For this review, take the finished solid that the model builds, in its own axes (mm). Face numbers are marked on the shaded views. A direction names the side the tool comes from. Round coordinates to 2 decimals unless told otherwise and drop trailing zeros. Order: outer loops, then holes, each group sorted by start corner. A loop starts at its lowest first (then second) coordinate and runs counter-clockwise, first axis right, second up.
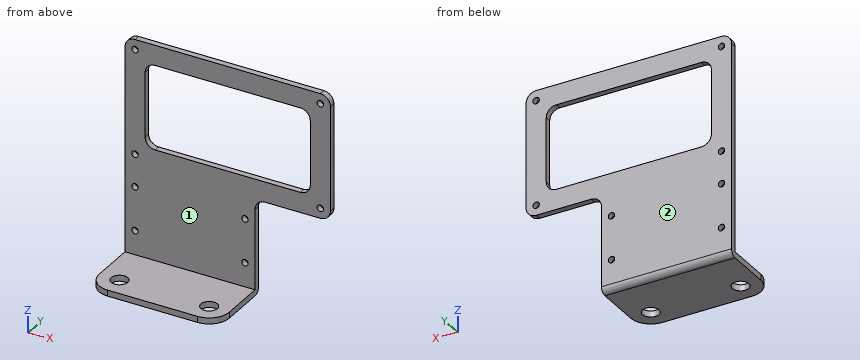
```python
from build123d import *

# Parameters (mm, degrees)
SKETCH_1_W          = 110
SKETCH_1_H          = 110
EXTRUDE_1_DEPTH     = 3
CUT_EXTRUDE_1_REACH = 79.84
SKETCH_2_R          = 1.6
CUT_EXTRUDE_2_REACH = 79.84
SKETCH_5_W          = 64.6
SKETCH_5_H          = 3
EXTRUDE_2_DEPTH     = 32
CUT_EXTRUDE_3_REACH = 129.079
SKETCH_6_R          = 4.1
CUT_EXTRUDE_4_REACH = 87.294
FILLET_1_R          = 5
FILLET_2_R          = 3
FILLET_3_R          = 10


with BuildPart() as part:
    # 草图1 → 凸台-拉伸1 (new body)
    with BuildSketch(Plane(origin=(0, 0, 0), x_dir=(1, 0, 0), z_dir=(0, 1, 0))):
        Rectangle(SKETCH_1_W, SKETCH_1_H)
    extrude(amount=EXTRUDE_1_DEPTH)

    # 草图2 → 切除-拉伸1 (cut, up to next)
    with BuildSketch(Plane(origin=(0, 3, 0), x_dir=(1, 0, 0), z_dir=(0, 1, 0)), mode=Mode.PRIVATE) as cut_extrude_1_sk1:
        with Locations(Location((-50, 40, 0), (0, 0, 270))):
            Circle(SKETCH_2_R)
    cut_extrude_1_tool1 = extrude(cut_extrude_1_sk1.sketch, amount=-CUT_EXTRUDE_1_REACH, mode=Mode.PRIVATE) & part.part
    # 草图2 → 切除-拉伸1 (cut, up to next)
    with BuildSketch(Plane(origin=(0, 3, 0), x_dir=(1, 0, 0), z_dir=(0, 1, 0)), mode=Mode.PRIVATE) as cut_extrude_1_sk2:
        with Locations(Location((4.6, 40, 0), (0, 0, 270))):
            Circle(SKETCH_2_R)
    cut_extrude_1_tool2 = extrude(cut_extrude_1_sk2.sketch, amount=-CUT_EXTRUDE_1_REACH, mode=Mode.PRIVATE) & part.part
    # 草图2 → 切除-拉伸1 (cut, up to next)
    with BuildSketch(Plane(origin=(0, 3, 0), x_dir=(1, 0, 0), z_dir=(0, 1, 0)), mode=Mode.PRIVATE) as cut_extrude_1_sk3:
        with Locations(Location((4.6, 18.2, 0), (0, 0, 270))):
            Circle(SKETCH_2_R)
    cut_extrude_1_tool3 = extrude(cut_extrude_1_sk3.sketch, amount=-CUT_EXTRUDE_1_REACH, mode=Mode.PRIVATE) & part.part
    # 草图2 → 切除-拉伸1 (cut, up to next)
    with BuildSketch(Plane(origin=(0, 3, 0), x_dir=(1, 0, 0), z_dir=(0, 1, 0)), mode=Mode.PRIVATE) as cut_extrude_1_sk4:
        with Locations(Location((-50, 18.2, 0), (0, 0, 270))):
            Circle(SKETCH_2_R)
    cut_extrude_1_tool4 = extrude(cut_extrude_1_sk4.sketch, amount=-CUT_EXTRUDE_1_REACH, mode=Mode.PRIVATE) & part.part
    # 草图2 → 切除-拉伸1 (cut, up to next)
    with BuildSketch(Plane(origin=(0, 3, 0), x_dir=(1, 0, 0), z_dir=(0, 1, 0)), mode=Mode.PRIVATE) as cut_extrude_1_sk5:
        with Locations(Location((-50, -50, 0), (0, 0, 270))):
            Circle(SKETCH_2_R)
    cut_extrude_1_tool5 = extrude(cut_extrude_1_sk5.sketch, amount=-CUT_EXTRUDE_1_REACH, mode=Mode.PRIVATE) & part.part
    # 草图2 → 切除-拉伸1 (cut, up to next)
    with BuildSketch(Plane(origin=(0, 3, 0), x_dir=(1, 0, 0), z_dir=(0, 1, 0)), mode=Mode.PRIVATE) as cut_extrude_1_sk6:
        with Locations(Location((42, -50, 0), (0, 0, 270))):
            Circle(SKETCH_2_R)
    cut_extrude_1_tool6 = extrude(cut_extrude_1_sk6.sketch, amount=-CUT_EXTRUDE_1_REACH, mode=Mode.PRIVATE) & part.part
    # 草图2 → 切除-拉伸1 (cut, up to next)
    with BuildSketch(Plane(origin=(0, 3, 0), x_dir=(1, 0, 0), z_dir=(0, 1, 0)), mode=Mode.PRIVATE) as cut_extrude_1_sk7:
        with Locations(Location((42, 2, 0), (0, 0, 270))):
            Circle(SKETCH_2_R)
    cut_extrude_1_tool7 = extrude(cut_extrude_1_sk7.sketch, amount=-CUT_EXTRUDE_1_REACH, mode=Mode.PRIVATE) & part.part
    # 草图2 → 切除-拉伸1 (cut, up to next)
    with BuildSketch(Plane(origin=(0, 3, 0), x_dir=(1, 0, 0), z_dir=(0, 1, 0)), mode=Mode.PRIVATE) as cut_extrude_1_sk8:
        with Locations(Location((-50, 2, 0), (0, 0, 270))):
            Circle(SKETCH_2_R)
    cut_extrude_1_tool8 = extrude(cut_extrude_1_sk8.sketch, amount=-CUT_EXTRUDE_1_REACH, mode=Mode.PRIVATE) & part.part
    add(cut_extrude_1_tool1.solids().sort_by_distance((-50, 3, -40))[0], mode=Mode.SUBTRACT)
    add(cut_extrude_1_tool2.solids().sort_by_distance((4.6, 3, -40))[0], mode=Mode.SUBTRACT)
    add(cut_extrude_1_tool3.solids().sort_by_distance((4.6, 3, -18.2))[0], mode=Mode.SUBTRACT)
    add(cut_extrude_1_tool4.solids().sort_by_distance((-50, 3, -18.2))[0], mode=Mode.SUBTRACT)
    add(cut_extrude_1_tool5.solids().sort_by_distance((-50, 3, 50))[0], mode=Mode.SUBTRACT)
    add(cut_extrude_1_tool6.solids().sort_by_distance((42, 3, 50))[0], mode=Mode.SUBTRACT)
    add(cut_extrude_1_tool7.solids().sort_by_distance((42, 3, -2))[0], mode=Mode.SUBTRACT)
    add(cut_extrude_1_tool8.solids().sort_by_distance((-50, 3, -2))[0], mode=Mode.SUBTRACT)

    # 草图3 → 切除-拉伸2 (cut, up to next)
    with BuildSketch(Plane(origin=(0, 3, 0), x_dir=(1, 0, 0), z_dir=(0, 1, 0)), mode=Mode.PRIVATE) as cut_extrude_2_sk1:
        Polygon((55, 17), (55, -55), (47, -55), (47, 7), (9.6, 7), (9.6, 55), (55, 55), align=None)
    cut_extrude_2_tool1 = extrude(cut_extrude_2_sk1.sketch, amount=-CUT_EXTRUDE_2_REACH, mode=Mode.PRIVATE) & part.part
    add(cut_extrude_2_tool1.solids().sort_by_distance((35.767105, 3, -20.802632))[0], mode=Mode.SUBTRACT)

    # 草图5 → 凸台-拉伸2 (add)
    with BuildSketch(Plane.XZ):
        with Locations((-22.7, -53.5)):
            Rectangle(SKETCH_5_W, SKETCH_5_H)
    extrude(amount=EXTRUDE_2_DEPTH)

    # 草图6 → 切除-拉伸3 (cut, up to next)
    with BuildSketch(Plane(origin=(0, 0, -55), x_dir=(-1, 0, 0), z_dir=(0, 0, -1)), mode=Mode.PRIVATE) as cut_extrude_3_sk1:
        with Locations((0.4, -22)):
            Circle(SKETCH_6_R)
    cut_extrude_3_tool1 = extrude(cut_extrude_3_sk1.sketch, amount=-CUT_EXTRUDE_3_REACH, mode=Mode.PRIVATE) & part.part
    # 草图6 → 切除-拉伸3 (cut, up to next)
    with BuildSketch(Plane(origin=(0, 0, -55), x_dir=(-1, 0, 0), z_dir=(0, 0, -1)), mode=Mode.PRIVATE) as cut_extrude_3_sk2:
        with Locations((45, -22)):
            Circle(SKETCH_6_R)
    cut_extrude_3_tool2 = extrude(cut_extrude_3_sk2.sketch, amount=-CUT_EXTRUDE_3_REACH, mode=Mode.PRIVATE) & part.part
    add(cut_extrude_3_tool1.solids().sort_by_distance((-0.4, -22, -55))[0], mode=Mode.SUBTRACT)
    add(cut_extrude_3_tool2.solids().sort_by_distance((-45, -22, -55))[0], mode=Mode.SUBTRACT)

    # 草图7 → 切除-拉伸4 (cut, up to next)
    with BuildSketch(Plane(origin=(0, 3, 0), x_dir=(1, 0, 0), z_dir=(0, 1, 0)), mode=Mode.PRIVATE) as cut_extrude_4_sk1:
        with BuildLine():
            Line((-40, -3), (32, -3))
            ThreePointArc((32, -3), (35.535533906, -4.464466094), (37, -8))
            Line((37, -8), (37, -40))
            ThreePointArc((37, -40), (35.535533906, -43.535533906), (32, -45))
            Line((32, -45), (-40, -45))
            ThreePointArc((-40, -45), (-43.535533906, -43.535533906), (-45, -40))
            Line((-45, -40), (-45, -8))
            ThreePointArc((-45, -8), (-43.535533906, -4.464466094), (-40, -3))
        make_face()
    cut_extrude_4_tool1 = extrude(cut_extrude_4_sk1.sketch, amount=-CUT_EXTRUDE_4_REACH, mode=Mode.PRIVATE) & part.part
    add(cut_extrude_4_tool1.solids().sort_by_distance((-4, 3, 24))[0], mode=Mode.SUBTRACT)

    # 圆角1
    fillet_1_edges = [part.edges().sort_by_distance(p)[0] for p in [
        (47, 1.5, 55),
        (47, 1.5, -7),
        (9.6, 1.5, -7),
        (-55, 1.5, 55),
    ]]
    fillet(fillet_1_edges, radius=FILLET_1_R)

    # 圆角2
    fillet_2_edges = [part.edges().sort_by_distance(p)[0] for p in [
        (-22.7, 3, -55),
    ]]
    fillet(fillet_2_edges, radius=FILLET_2_R)

    # 圆角3
    fillet_3_edges = [part.edges().sort_by_distance(p)[0] for p in [
        (9.6, -32, -53.5),
        (-55, -32, -53.5),
    ]]
    fillet(fillet_3_edges, radius=FILLET_3_R)


solid = part.part
```
Q1. Take a section at D-D, the plane y = -3.5. State the section outline as (x, z) points.
Q2. Clearance check with flat-ended pins moving along their axes: pin 1 (4 mm diameter, centred on x = -50, z = 50, fed in from +Y); pin 2 (5 mm diameter, centred on x = 4.6, z = -40, fed in from -Y); pin 3 (2.5 mm diameter, centred on x = 42, z = -2, fed in from -Y); pin 4 (16 mm diameter, centred on x = -8, y = -11.5, fed in from +Z). State where each tip first meets the part, or that it passes through.
Q3. Tool access review of the marked faces 1 and 2: name each direction out of +Z, -Z, +X, -X, +Y, -Y from which nothing blocks a thin tool from reaching the whole face with its end or side.
Q4. Take a section at A-A, the plane z = 17. State the section outline as (x, y) points, plus the area to 3 significant figures.
Q5. Wall thickness on line 1 (X direction, y = 2, z = -2); line 2 (X direction, y = 2, z = -40); line 3 (Z direction, x = 4, y = 2): over which ranges is each line inside the solid? List them lowest first.
Q6. Take a section at B-B, the plane x = -19. State the section outline as (y, z) points.
Q7. Take a section at C-C, the plane z = -40. State the section outline as (x, y) points.
Working result:
1. outline: (-55, -55) - (9.6, -55) - (9.6, -52) - (-55, -52) - close
2. pin 1: stops at y = 3
2. pin 2: stops at y = 0
2. pin 3: passes through
2. pin 4: stops at z = -52
3. face 1: +Z, +X, -X, -Y
3. face 2: +Z, -Z, +X, -X, +Y
4. outline: (-55, 0) - (-45, 0) - (-45, 3) - (-55, 3) - close; (37, 0) - (47, 0) - (47, 3) - (37, 3) - close
4. area: 60.0 mm2
5. line 1: x = -55 to -51.6, -48.4 to 40.4, 43.6 to 47
5. line 2: x = -55 to -51.6, -48.4 to 3, 6.2 to 9.6
5. line 3: z = -54.24 to -41.48, -38.52 to -19.68, -16.72 to 3, 45 to 55
6. outline: (-32, -55) - (0, -55) arc R3 ccw to (3, -52) - (3, 3) - (0, 3) - (0, -52) - (-32, -52) - close; (0, 45) - (3, 45) - (3, 55) - (0, 55) - close
7. outline: (-55, 0) - (-51.6, 0) - (-51.6, 3) - (-55, 3) - close; (-48.4, 0) - (3, 0) - (3, 3) - (-48.4, 3) - close; (6.2, 0) - (9.6, 0) - (9.6, 3) - (6.2, 3) - close
